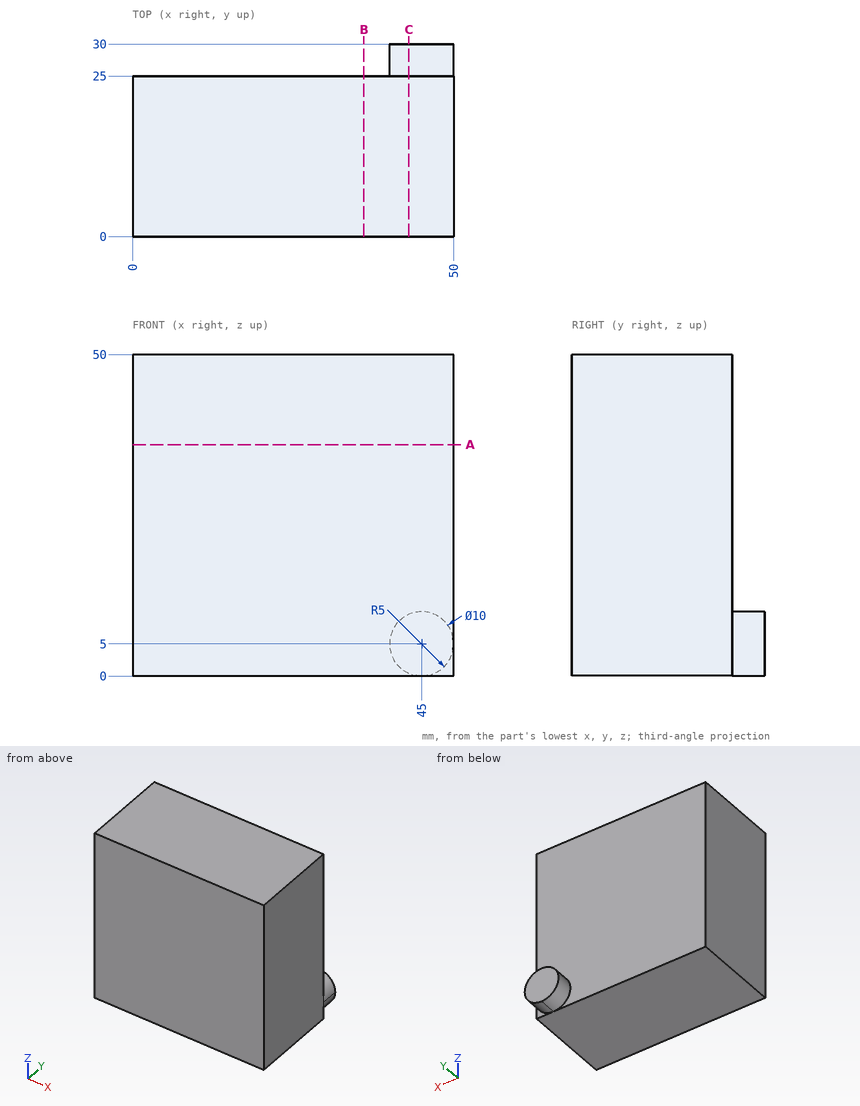
Geometry: see drawing. Coordinates: mm, zero at the bounding-box minimum. Round coordinates to 2 decimals unless told otherwise and drop trailing zeros. Write each loop counter-clockwise with the first axis right and the second up, starting at its lowest first coordinate (ties: lowest second). Pieces come first, ordered by that corner, then holes.
1) Cut plane A-A (z = 36). Return the cut outline in (x, y).
2) Cut plane C-C (x = 43). Return the cut outline in (y, z), then the cut area to 3 significant figures.
3) Ray query, L1, parallel to Y at x = 23.5, z = 9; L2, parallel to Z at x = 44.5, y = 27.25; L3, parallel to Z at x = 48, y = 26. Return the intervals inside material, ascending.
4) Contact query for a flat-ended pin moving along its axis: P1, Ø25, axis at x = 23, z = 23.5, coming from the +Y side. Output: stop coordinate, or through.
5) Cut plane B-B (x = 36). Return the cut outline in (y, z), then the cut area to 3 significant figures.
Geometry says:
1. outline: (0, 0) - (50, 0) - (50, 25) - (0, 25) - close
2. outline: (0, 0) - (25, 0) - (25, 0.42) - (30, 0.42) - (30, 9.58) - (25, 9.58) - (25, 50) - (0, 50) - close
2. area: 1,300 mm2
3. L1: y = 0 to 25
3. L2: z = 0.03 to 9.97
3. L3: z = 1 to 9
4. P1: stops at y = 25
5. outline: (0, 0) - (25, 0) - (25, 50) - (0, 50) - close
5. area: 1,250 mm2
